Geometry check sheet. Reference: drawing and pictorial views, mm from the part's lowest x, y, z. Give positions to 0.01 mm unless a question says otherwise; leave off trailing zeros. Write each loop counter-clockwise with the first axis right and the second up, starting at its lowest first coordinate (ties: lowest second). Pieces come first, ordered by that corner, then holes. Notation, with made-up numbers: (-36, -36) -> (12, -36) arc R32 ccw to (12, -2) -> close; hole circle Ø1 at (2, -34.75). An arc over 180 degrees is marked (long way). Return JSON: item names as keys, results as strings.
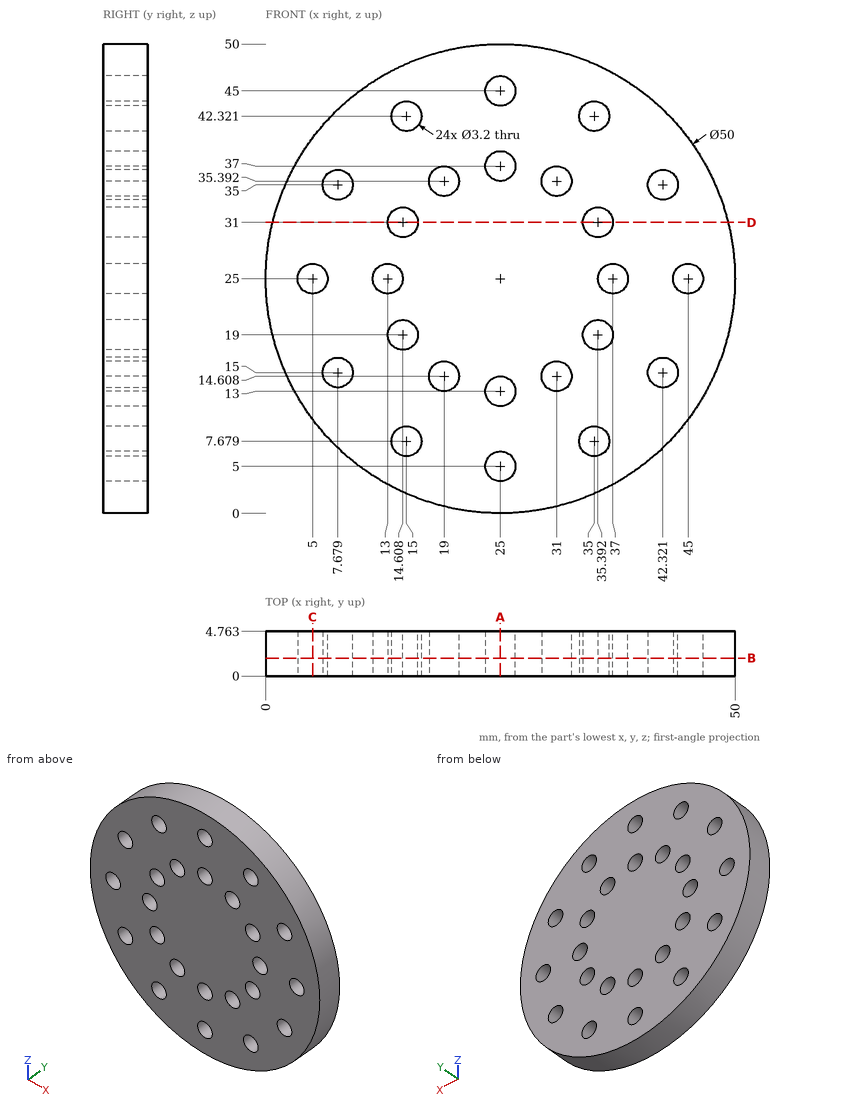
(1) Cross-section at D-D on z = 31. Enter the section's corners in (x, y).
Reply:
{"outline": "(0.73, 0) -> (13.01, 0) -> (13.01, 4.76) -> (0.73, 4.76) -> close; (16.21, 0) -> (33.79, 0) -> (33.79, 4.76) -> (16.21, 4.76) -> close; (36.99, 0) -> (49.27, 0) -> (49.27, 4.76) -> (36.99, 4.76) -> close"}
(2) Cross-section at B-B on y = 1.9. State how many separate pieces and enclosed holes the cut face has, then the cut area to 3 significant figures.
Reply:
{"separate pieces": "1", "enclosed holes": "24", "area": "1,770 mm^2"}
(3) Thickness scan on L1, parallel to Z at x = 18.5, y = 2.05; L2, parallel to Z at x = 32, y = 1 (1 decimal); L3, parallel to Z at x = 24, y = 3.85. Record the ranges inside material, lowest first.
Reply:
{"L1": "0.86 to 13.09, 16.13 to 33.87, 36.91 to 49.14", "L2": "1 to 13.4, 15.9 to 34.1, 36.6 to 49", "L3": "0.02 to 3.75, 6.25 to 11.75, 14.25 to 35.75, 38.25 to 43.75, 46.25 to 49.98"}
(4) Cross-section at A-A on x = 25. Enter the section's corners in (y, z).
Reply:
{"outline": "(0, 0) -> (4.76, 0) -> (4.76, 3.4) -> (0, 3.4) -> close; (0, 6.6) -> (4.76, 6.6) -> (4.76, 11.4) -> (0, 11.4) -> close; (0, 14.6) -> (4.76, 14.6) -> (4.76, 35.4) -> (0, 35.4) -> close; (0, 38.6) -> (4.76, 38.6) -> (4.76, 43.4) -> (0, 43.4) -> close; (0, 46.6) -> (4.76, 46.6) -> (4.76, 50) -> (0, 50) -> close"}
(5) Depth check by flat-ended pin: pin 1 Ø1 at (x, y) = (21.5, 1) entering from +Z. Enter the tip coordinate at first touch or a pass-through.
Reply:
{"pin 1": "z = 49.82"}
(6) Cross-section at C-C on x = 5. Enter the section's corners in (y, z), then the cut area to 3 significant figures.
Reply:
{"outline": "(0, 10) -> (4.76, 10) -> (4.76, 23.4) -> (0, 23.4) -> close; (0, 26.6) -> (4.76, 26.6) -> (4.76, 40) -> (0, 40) -> close", "area": "128 mm^2"}
